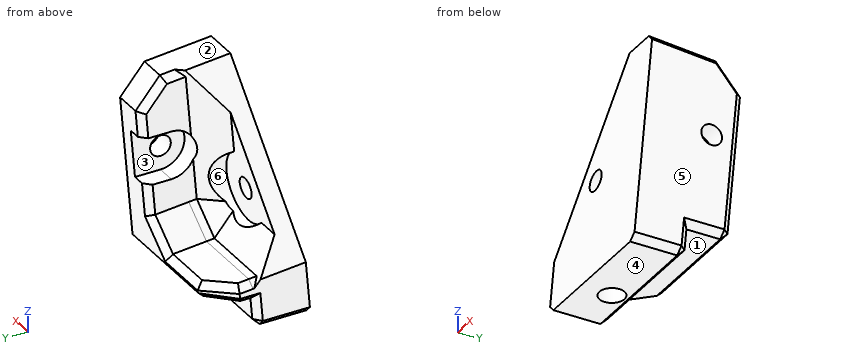
from build123d import *
from OCP.BRepFilletAPI import BRepFilletAPI_MakeChamfer

# Parameters (mm, degrees)
BOSS_EXTRUDE3_DEPTH             = 12.7
CUT_EXTRUDE1_DEPTH              = 2446.156245266122
CUT_EXTRUDE2_DEPTH              = 25.4
BOSS_EXTRUDE4_DEPTH             = 9.525
BOSS_EXTRUDE5_START             = -133.985000001
BOSS_EXTRUDE5_DEPTH             = 34.925
CUT_EXTRUDE3_REACH              = 2445.46
SKETCH12_W                      = 34.925000000000026
SKETCH12_H                      = 0.3325309889783057
CHAMFER4_SIZE                   = 6.35
CHAMFER5_SIZE                   = 1.5875
CHAMFER5_SIZE2                  = 1.7463498023569755
CHAMFER5_SIZE2_2                = 1.7463498023569135
CHAMFER5_SIZE2_3                = 1.695194438361193
CUT_EXTRUDE5_START              = 10.8585
CUT_EXTRUDE5_DEPTH              = 10.8585
F_8_START                       = -200.342016287
F_8_CLEARANCE_HOLE1_2_OUTLINE_W = 7
F_8_CLEARANCE_HOLE1_2_OUTLINE_H = 7
F_8_CLEARANCE_HOLE1_2_DEPTH     = 0.279842574
F_8_CLEARANCE_HOLE2_D           = 4.9149
CUT_EXTRUDE6_REACH              = 253.711
SKETCH24_R                      = 7.937499999999993


with BuildPart() as part:
    # Sketch6 → Boss-Extrude3 (new body)
    with BuildSketch(Plane(origin=(2.311843e-11, -2425.8151689885194, 212.23132709558422), x_dir=(1, 9.46e-15, -8.3e-16), z_dir=(9.493905125025943e-15, -0.9961946980917503, 0.08715574274760324))):
        Polygon((-99.0600000006817, -213.04201628669756), (-133.9850000006817, -213.04201628669756), (-133.9850000006817, -200.34201628669757), (-108.5850000006817, -162.24201628669755), (-99.0600000006817, -162.24201628669755), align=None)
    extrude(amount=-BOSS_EXTRUDE3_DEPTH)

    # Sketch7 → Cut-Extrude1 (cut, through all)
    with BuildSketch(Plane.ZY.offset(133.9850000006817)):
        Polygon((-2.4964e-13, -2444.383004154433), (0, -2431.6344922176327), (-1.1068779328950917, -2431.7313314886683), align=None)
    extrude(amount=-CUT_EXTRUDE1_DEPTH, mode=Mode.SUBTRACT)

    # Sketch8 → Cut-Extrude2 (cut)
    with BuildSketch(Plane.ZY.offset(133.9850000006817)):
        Polygon((50.219283386547545, -2435.5274069898373), (12.26426538925185, -2438.848040788521), (11.544794732870468, -2430.6244535557735), (49.49981273016616, -2427.30381975709), align=None)
    extrude(amount=-CUT_EXTRUDE2_DEPTH, mode=Mode.SUBTRACT)

    # Sketch10 → Boss-Extrude4 (add, through all)
    with BuildSketch(Plane.ZY.offset(108.58500000067501)):
        Polygon((49.499812730166134, -2427.3038197570895), (11.544794732870441, -2430.624453555773), (10.711465212786628, -2421.099453555773), (48.66648321008233, -2417.7788197570894), align=None)
    extrude(amount=-BOSS_EXTRUDE4_DEPTH)

    # Boss-Extrude5: read off the stored shape, not the designer's step
    # Boss-Extrude5 outline → Boss-Extrude5 (add)
    with BuildSketch(Plane.YZ.offset(BOSS_EXTRUDE5_START)):
        Polygon((-2420.768187948, 10.682483227), (-2430.624453556, 11.544794733), (-2431.031161645, 6.8961), (-2421.099453556, 6.8961), align=None)
    extrude(amount=BOSS_EXTRUDE5_DEPTH)

    # Sketch12 → Cut-Extrude3 (cut, up to next)
    with BuildSketch(Plane(origin=(0, -17.46095723301537, -199.5796544297948), x_dir=(1, 0, 0), z_dir=(0, 0.0871557427475931, 0.9961946980917512)), mode=Mode.PRIVATE) as cut_extrude3_sk1:
        with Locations((-116.52250000065857, -2412.653739397144)):
            Rectangle(SKETCH12_W, SKETCH12_H)
    cut_extrude3_tool1 = extrude(cut_extrude3_sk1.sketch, amount=-CUT_EXTRUDE3_REACH, mode=Mode.PRIVATE) & part.part
    add(cut_extrude3_tool1.solids().sort_by_distance((-116.5225, -2420.933821, 10.696974))[0], mode=Mode.SUBTRACT)

    # Chamfer4
    chamfer4_edges = [part.edges().sort_by_distance(p)[0] for p in [
        (-108.58500000065862, -2437.1877238891802, 31.241774387899785),
        (-108.58500000065875, -2425.8619535557737, 11.1281299728286),
        (-121.28500000065863, -2438.848040788522, 12.26426538925195),
        (-103.82250000065878, -2417.7788197570903, 48.6664832100824),
        (-133.98500000065857, -2421.266354157439, 8.803782606393371),
    ]]
    chamfer(chamfer4_edges, length=CHAMFER4_SIZE)

    # Chamfer5: one chamfer whose edges measure the first distance from different faces: ONE call of the kernel's chamfer builder (chamfer() names one face for all edges)
    chamfer5_edges_1 = [part.edges().sort_by_distance(p)[0] for p in [
        (-111.76000000038354, -2420.822734072567, 13.874383379035507),
        (-99.0600000006587, -2431.3328269313633, 3.4480500000041445),
        (-99.06000000065865, -2438.0087481860337, -4.5e-14),
        (-133.98500000065866, -2438.008748186034, -1.396e-14),
        (-133.98500000065872, -2431.332826931364, 3.448050000004116),
        (-133.985000001, -2429.419336186252, 6.8961),
        (-99.060000001, -2426.232208202052, 6.8961),
        (-108.58500000065878, -2419.43913665644, 29.688974211344913),
        (-99.06000000075693, -2419.8827567413205, 24.618373438599672),
        (-121.28500000051437, -2421.099453555774, 10.711465212786711),
        (-133.985000001, -2429.024871722332, 11.404849456074741),
        (-130.81000000070145, -2424.262371722282, 10.988184695738429),
        (-99.06000000065865, -2432.030074256415, 49.91330641979526),
        (-108.5850000006587, -2426.6531133734643, 49.44288329831503),
        (-108.58500000065877, -2421.218457406756, 45.780284526864456),
        (-99.06000000065876, -2421.2184574067555, 45.78028452686439),
    ]]
    chamfer5_edges_2 = [part.edges().sort_by_distance(p)[0] for p in [
        (-116.52250000065871, -2431.634492217634, 9.642e-14),
    ]]
    chamfer5_side_2 = [part.faces().sort_by_distance(p)[0] for p in [
        (-116.52250000065865, -2438.008748186034, -2.841e-14),
    ]]
    chamfer5_edges_3 = [part.edges().sort_by_distance(p)[0] for p in [
        (-113.34750000082943, -2421.433254759104, 6.896099999999999),
    ]]
    chamfer5_side_3 = [part.faces().sort_by_distance(p)[0] for p in [
        (-115.53645576803177, -2426.404038617734, 6.8961),
    ]]
    chamfer5_edges_4 = [part.edges().sort_by_distance(p)[0] for p in [
        (-130.81000000070134, -2424.6203827433465, 6.8961),
    ]]
    chamfer5_side_4 = [part.faces().sort_by_distance(p)[0] for p in [
        (-130.8815677895093, -2424.512945541763, 8.945261119766531),
    ]]
    chamfer5 = BRepFilletAPI_MakeChamfer(part.part.solid().wrapped)
    for e in chamfer5_edges_1:
        chamfer5.Add(CHAMFER5_SIZE, e.wrapped)
    for e in chamfer5_edges_2:
        chamfer5.Add(CHAMFER5_SIZE, CHAMFER5_SIZE2, e.wrapped, chamfer5_side_2[0].wrapped)  # the first distance lies on this face
    for e in chamfer5_edges_3:
        chamfer5.Add(CHAMFER5_SIZE, CHAMFER5_SIZE2_2, e.wrapped, chamfer5_side_3[0].wrapped)  # the first distance lies on this face
    for e in chamfer5_edges_4:
        chamfer5.Add(CHAMFER5_SIZE, CHAMFER5_SIZE2_3, e.wrapped, chamfer5_side_4[0].wrapped)  # the first distance lies on this face
    add(Compound.cast(chamfer5.Shape()), mode=Mode.REPLACE)

    # Sketch14 → CBORE for #8 Pan Head Machine Screw1 (revolve, cut)
    with BuildSketch(Plane(origin=(-108.58500000065874, -2425.9412416479745, 30.25783468724938), x_dir=(5.9e-16, 0, 1), z_dir=(-6.7e-15, 1, 0))):
        Polygon((0, 0), (-2.33e-15, 9.525000000000226), (2.4574499999999975, 9.525000000000226), (2.4574499999999997, 4.508499999999999), (5.715, 4.508499999999999), (5.715, 0), align=None)
    revolve(axis=Axis((-114.93500000065873, -2425.9412416479745, 30.257834687249385), (1, 7.96e-15, -5.9e-16)), mode=Mode.SUBTRACT)

    # Sketch16 → Cut-Extrude5 (cut)
    with BuildSketch(Plane.ZY.offset(104.07650000065875).offset(CUT_EXTRUDE5_START)):
        with BuildLine():
            Line((35.972834687249275, -2425.9412416479745), (35.972834687249254, -2417.8454644621274))
            Line((35.972834687249254, -2417.8454644621274), (24.542834687249364, -2418.845459886228))
            Line((24.542834687249364, -2418.845459886228), (24.542834687249364, -2425.9412416479745))
            ThreePointArc((24.542834687249364, -2425.9412416479745), (30.257834687249318, -2431.6562416479746), (35.972834687249275, -2425.9412416479745))
        make_face()
    extrude(amount=-CUT_EXTRUDE5_DEPTH, mode=Mode.SUBTRACT)

    # Sketch18 → Hole1 (revolve, cut)
    with BuildSketch(Plane(origin=(-121.28500000067221, -2436.8657251652107, -4.765035e-11), x_dir=(0, 1, 1.96e-14), z_dir=(1, 0, -8.3e-16))):
        Polygon((0, 0), (0, 4.6989999999999945), (2.870200000000013, 4.6989999999999945), (2.9972000000000123, 0), align=None)
    revolve(axis=Axis((-121.28500000067213, -2436.865725165213, 109.99999999995235), (-8.3e-16, 1.895e-14, -1)), mode=Mode.SUBTRACT)

    # #8 Clearance Hole1: read off the stored shape, not the designer's step
    # #8 Clearance Hole1 outline → #8 Clearance Hole1 (revolve, cut)
    with BuildSketch(Plane(origin=(-121.285000001, -2436.865725165, 0), x_dir=(1, 0, 0), z_dir=(0, -1, 0))):
        Polygon((2.45745, 4.699), (2.45745, 11.711826423), (1.590785336, 12.232571089), (0, 12.232571089), (0, 4.699), align=None)
    revolve(axis=Axis((-121.285000001, -2436.865725165, 0), (0, 0, 1)), mode=Mode.SUBTRACT)

    # 8 Clearance Hole1 2 outline → 8 Clearance Hole1 2 (add)
    with BuildSketch(Plane(origin=(0, 0, 0), x_dir=(1, 0, 0), z_dir=(0, 0.08715574274759312, 0.9961946980917512)).offset(F_8_START)):
        with Locations((-121.50000000000001, -2428.5)):
            Rectangle(F_8_CLEARANCE_HOLE1_2_OUTLINE_W, F_8_CLEARANCE_HOLE1_2_OUTLINE_H)
    extrude(amount=F_8_CLEARANCE_HOLE1_2_DEPTH)

    # #8 Clearance Hole2 (through all)
    with Locations(Plane(origin=(3.101414e-11, -2425.8151689885194, 212.23132709558124), x_dir=(-1, -1.269e-14, 1.11e-15), z_dir=(1.2736388665441791e-14, -0.9961946980917505, 0.08715574274760202))):
        with Locations((118.639166667, 188.435766287)):
            Hole(F_8_CLEARANCE_HOLE2_D / 2)

    # Sketch24 → Cut-Extrude6 (cut, up to next)
    with BuildSketch(Plane(origin=(2.307623e-11, -2421.3870835555053, 211.84391981904722), x_dir=(1, 9.46e-15, -8.3e-16), z_dir=(-9.493905125025941e-15, 0.9961946980917512, -0.08715574274759331)), mode=Mode.PRIVATE) as cut_extrude6_sk1:
        with Locations((-118.6391666673483, 188.43576628667344)):
            Circle(SKETCH24_R)
    cut_extrude6_tool1 = extrude(cut_extrude6_sk1.sketch, amount=CUT_EXTRUDE6_REACH, mode=Mode.PRIVATE) & part.part
    add(cut_extrude6_tool1.solids().sort_by_distance((-118.639167, -2437.810343, 24.125209))[0], mode=Mode.SUBTRACT)


solid = part.part
Geometry: final body of the model. Coordinates: model frame, mm. Face numbers are marked on the shaded views. A direction names the side the tool comes from. Coordinates: 2 decimals unless noted, no trailing zeros. Loops run counter-clockwise (first coordinate to the right, second up) from the corner with the lowest first, then second, coordinate; pieces in that order, holes last. Notation, with made-up numbers: (74.5, 22.5) - (107.5, 22.5) arc R18 ccw to (107.5, 49.5) - close; hole circle Ø6 at (-6, -11). An arc over 180 degrees is marked (long way). Put each result on its own line as item: value. Start each with the question number.
Q1. Cut plane A-A, the plane y = -2427. Return loops of the section in (x, z) (1 decimal).
Q2. Cut plane B-B, the plane x = -105. Return loops of the section in (y, z) (1 decimal), and give its area (3 significant figures).
Q3. Set-up query: the marked faces 1, 2 and 3. Return all of +Z, -Z, +X, -X, +Y, -Y with unobstructed straight access to the full face (end or side cutting, diameter ignored); none if empty.
Q4. Line query: line 1 (X direction, y = -2422.75, z = 28); line 2 (Z direction, x = -105, y = -2427.25); line 3 (X direction, y = -2442.25, z = 24). Output: solid intervals per line, ascending.
Q5. Pin query (flat end, axial travel): pin 1 Ø8.5 at (y, z) = (-2428.5, 20.5) entering from -X; pin 2 Ø5.5 at (x, y) = (-121.29, -2436.87) entering from -Z; pin 3 Ø1.7 at (x, y) = (-121.5, -2436.5) entering from -Z. Return the tip coordinate at first contact, or that it passes through.
Q6. Pull-direction query (Z, two-part tool) for the marked faces 4, 5 and 6; classes: released by +Z, released by -Z, zero draft, split by the parting line, or undercut.
Q7. Cut plane D-D, the plane x = -125.5. Return loops of the section in (y, z), and give its area (3 significant figures).
Q8. Cut plane C-C, the plane z = 44.5. Return loops of the section in (x, y) (1 decimal).
Filled sheet:
1. outline: (-133.4, 9.6) - (-133.3, 8.5) - (-130.8, 6.9) - (-100.6, 6.9) - (-99.1, 8.5) - (-99.1, 28) - (-104.1, 28) - (-104.1, 24.6) - (-108.6, 24.6) - (-108.6, 17.6) - (-114.9, 11.2) - (-131.3, 11.2) - close; (-108.6, 35.9) - (-104.1, 35.9) - (-104.1, 32.5) - (-99.1, 32.5) - (-99.1, 47.9) - (-100.6, 49.5) - (-107, 49.5) - (-108.6, 47.9) - close
2. outline: (-2444.4, 0) - (-2433.2, 0) - (-2431.5, 1.7) - (-2431, 6.9) - (-2423, 6.9) - (-2421.3, 8.6) - (-2419.9, 24.5) - (-2425.9, 24.5) arc R5.7 cw to (-2425.9, 36) - (-2418.9, 36) - (-2418.3, 42.3) - (-2424.1, 49.2) - (-2440, 50.6) - close
2. area: 894 mm²
3. face 1: -Z, +X, -X, +Y
3. face 2: +Z, +X, -X, +Y
3. face 3: -X, +Y
4. line 1: -104.08 to -99.06
4. line 2: 6.9 to 24.69, 35.82 to 49.5
4. line 3: -126.39 to -121.04, -116.24 to -99.06
5. pin 1: x = -110.08
5. pin 2: z = 4.7
5. pin 3: z = 11.98
6. face 4: released by -Z
6. face 5: zero draft
6. face 6: undercut
7. outline: (-2444.38, 0) - (-2433.22, 0) - (-2431.48, 1.74) - (-2431.03, 6.9) - (-2423.02, 6.9) - (-2421.28, 8.64) - (-2421.24, 9.13) - (-2422.68, 10.85) - (-2432.52, 11.71) - (-2438.29, 18.59) - (-2437.74, 24.94) - (-2442.17, 25.33) - close
7. area: 268 mm²
8. outline: (-112.7, -2440.5) - (-99.1, -2440.5) - (-99.1, -2422.2) - (-100.6, -2420.1) - (-107, -2420.1) - (-108.6, -2422.2) - (-108.6, -2429.7) - (-112.3, -2433.3) - close
